Verification items for the finished model (mm, model axes). Round coordinates to 2 decimals unless told otherwise and drop trailing zeros. Loops run counter-clockwise (first coordinate to the right, second up) from the corner with the lowest first, then second, coordinate; pieces in that order, holes last. Notation, with made-up numbers: (-0.75, 86) -> (14.25, 86) arc R21 ccw to (14.25, 117) -> close; hole circle Ø4 at (71, 59.5). An arc over 180 degrees is marked (long way). Use a Markdown table: item, result. Add a question column.
```python
from build123d import *

# Parameters (mm, degrees)
CUT_EXTRUDE1_DEPTH = 23.5


with BuildPart() as part:
    # Sketch1 → Revolve1 (revolve)
    with BuildSketch(Plane.XY, mode=Mode.PRIVATE) as revolve1_sk:
        Polygon((-22.25, 0.384913229), (-0.783076171, 43.5), (-0.01, 43.115086771), (-21.476923829, 0), align=None)
    revolve(revolve1_sk.sketch.rotate(Axis((0, 0, 0), (0, 1, 0)), 270), axis=Axis((0, 0, 0), (0, 1, 0)))

    # Sketch3 → Cut-Extrude1 (cut)
    with BuildSketch(Plane(origin=(0, 43.5, 0), x_dir=(-1, 0, 0), z_dir=(0, -1, 0))):
        Polygon((-20.4318, -0.4318), (-20.4318, 0.4318), (-0.4318, 0.4318), (-0.4318, 20.4318), (0.4318, 20.4318), (0.4318, 0.4318), (20.4318, 0.4318), (20.4318, -0.4318), (0.4318, -0.4318), (0.4318, -20.4318), (-0.4318, -20.4318), (-0.4318, -0.4318), align=None)
    extrude(amount=CUT_EXTRUDE1_DEPTH, mode=Mode.SUBTRACT)


solid = part.part
```
1) Sectioned sample at A-A on y = 22.5. Enter the section's corners in (x, z).
2) Release check for a two-part mould opening along Z. For faces 1 (the face through (-2.7, 27.03, -8.57)), 2 (the face through (6.4, 30.9, 0.432)), 3 (the face through (-0.432, 30.9, 6.4)), 4 (the face through (-2.66, 25.32, -8.46)) record: released by +Z, released by -Z, zero draft, split by the parting line, or undercut.
3) Thickness scan on line 1 (Z direction, x = -2, y = 18); line 2 (X direction, y = 15.5, z = -5); line 3 (X direction, y = 15.5, z = 7). Record the ranges inside material, lowest first.
4) Sectioned sample at C-C on y = 32.5. Enter the section's corners in (x, z).
5) Sectioned sample at D-D on y = 3. Enter the section's corners in (x, z).
6) Go/stop test with flat-tipped pins: pin 1 (0.7 mm diameter, centred on x = 12, z = 0, fed in from +Y); pin 2 (1.5 mm diameter, centred on x = 2.5, z = 6, fed in from -Y); pin 3 (13 mm diameter, centred on y = 34, z = 4, fed in from +X); pin 4 (6 mm diameter, centred on y = 37, z = 9, fed in from -X). Record where each tip stops, or that it passes through.
7) Sectioned sample at B-B on y = 9. Enter the section's corners in (x, z), then the cut area to 3 significant figures.
Geometry results:
| question | item | result |
|---|---|---|
| 1 | outline | (-11.23, -0.43) arc R11.24 ccw to (-0.43, -11.23) -> (-0.43, -10.27) arc R10.27 cw to (-10.27, -0.43) -> close; (-11.23, 0.43) -> (-10.27, 0.43) arc R10.27 cw to (-0.43, 10.27) -> (-0.43, 11.23) arc R11.24 ccw to start; (0.43, -11.23) arc R11.24 ccw to (11.23, -0.43) -> (10.27, -0.43) arc R10.27 cw to (0.43, -10.27) -> close; (0.43, 10.27) arc R10.27 cw to (10.27, 0.43) -> (11.23, 0.43) arc R11.24 ccw to (0.43, 11.23) -> close |
| 2 | face 1 | split by the parting line |
| 2 | face 2 | undercut |
| 2 | face 3 | zero draft |
| 2 | face 4 | undercut |
| 3 | line 1 | -13.33 to -12.35, 12.35 to 13.33 |
| 3 | line 2 | -13.85 to -12.82, 12.82 to 13.85 |
| 3 | line 3 | -12.95 to -11.85, 11.85 to 12.95 |
| 4 | outline | (-6.25, -0.43) arc R6.26 ccw to (-0.43, -6.25) -> (-0.43, -5.28) arc R5.3 cw to (-5.28, -0.43) -> close; (-6.25, 0.43) -> (-5.28, 0.43) arc R5.3 cw to (-0.43, 5.28) -> (-0.43, 6.25) arc R6.26 ccw to start; (0.43, -6.25) arc R6.26 ccw to (6.25, -0.43) -> (5.28, -0.43) arc R5.3 cw to (0.43, -5.28) -> close; (0.43, 5.28) arc R5.3 cw to (5.28, 0.43) -> (6.25, 0.43) arc R6.26 ccw to (0.43, 6.25) -> close |
| 5 | outline | circle Ø41.9 at (0, 0); hole circle Ø39.97 at (0, 0) |
| 6 | pin 1 | y = 20 |
| 6 | pin 2 | y = 28.57 |
| 6 | pin 3 | x = 8.37 |
| 6 | pin 4 | through |
| 7 | outline | circle Ø35.92 at (0, 0); hole circle Ø33.99 at (0, 0) |
| 7 | area | 106 mm^2 |
